```python
from build123d import *

# Parameters (mm, degrees)
SKETCH1_R           = 1
BOSS_EXTRUDE1_DEPTH = 2


with BuildPart() as part:
    # Sketch1 → Boss-Extrude1 (new body)
    with BuildSketch(Plane.XY):
        with BuildLine():
            Line((5.111751732, -19.659180157), (6, -22.203603311))
            ThreePointArc((6, -22.203603311), (0, 23), (-6, -22.203603311))
            Line((-6, -22.203603311), (-5.111751732, -19.659180157))
            ThreePointArc((-5.111751732, -19.659180157), (-5.690422868, -17.488375796), (-7.921535407, -17.224958453))
            ThreePointArc((-7.921535407, -17.224958453), (-10.119267773, -17.659121233), (-12.205757776, -16.843594198))
            ThreePointArc((-12.205757776, -16.843594198), (0, 19), (12.205757776, -16.843594198))
            ThreePointArc((12.205757776, -16.843594198), (10.119267773, -17.659121233), (7.921535407, -17.224958453))
            ThreePointArc((7.921535407, -17.224958453), (5.690422868, -17.488375796), (5.111751732, -19.659180157))
        make_face()
        with Locations((-7, -19)):
            Circle(SKETCH1_R, mode=Mode.SUBTRACT)
        with Locations((7, -19)):
            Circle(SKETCH1_R, mode=Mode.SUBTRACT)
    extrude(amount=BOSS_EXTRUDE1_DEPTH)


solid = part.part
```
Source: CAD feature listing. Evaluate the final solid. Frame: model axes, mm. A direction names the side the tool comes from. Give positions to 0.01 mm unless a question says otherwise; leave off trailing zeros. Loops run counter-clockwise (first coordinate to the right, second up) from the corner with the lowest first, then second, coordinate; pieces in that order, holes last. Notation, with made-up numbers: M -38,55 L -32,55 A13 ccw -32,61 Z; hole C -11,89 d3. An arc over 180 degrees is marked long. Put each result on its own line as item: value.
Q1. Section A-A (y = -6). Return the cut outline in (x, z).
Response values:
outline: M -22.2,0 L -19.36,0 L -19.36,2 L -22.2,2 Z; M 19.36,0 L 22.2,0 L 22.2,2 L 19.36,2 Z
Q2. Mould query, pull axis Y, two halves, no side actions, for faces 4 (the cylindrical face through (-0.696, 18.988, 0.986)), 5 (the flat face through (-5.562, -20.949, 0.986)), 6 (the cylindrical face through (10.151, -17.656, 0.986)), 7 (the flat face through (3, 19, 0)). Classes: released by +Y, released by -Y, zero draft, split by the parting line, or undercut.
Response values:
face 4: undercut
face 5: released by -Y
face 6: undercut
face 7: zero draft
Q3. Section D-D (z = 0.35). Return the cut outline in (x, y), and give its area (3 significant figures).
Response values:
outline: M -12.21,-16.84 A20 cw long 12.21,-16.84 A4 cw 7.92,-17.22 A2 ccw 5.11,-19.66 L 6,-22.2 A23 ccw long -6,-22.2 L -5.11,-19.66 A2 ccw -7.92,-17.22 A4 cw Z; hole C -7,-19 d2; hole C 7,-19 d2
area: 397 mm²
Q4. Line query: probe 1 along Y at (x, z) = (-7, 0.7) (3 decimals); probe 2 along X at (y, z) = (-13.5, 1.35); probe 3 along X at (y, z) = (5, 0.1). Output: solid intervals per line, ascending. Write a range as [from, to].
Response values:
probe 1: y = [-21.909, -20], [-18, -17], [17.735, 21.909]
probe 2: x = [-18.62, -15.61], [15.61, 18.62]
probe 3: x = [-22.45, -19.08], [19.08, 22.45]
Q5. Section B-B (x = -14). Return the cut outline in (y, z), and give its area (3 significant figures).
Response values:
outline: M -18.25,0 L -15.28,0 L -15.28,2 L -18.25,2 Z; M 13.28,0 L 18.25,0 L 18.25,2 L 13.28,2 Z
area: 15.9 mm²
Q6. Pin query (flat end, axial travel): P1, Ø2, axis at x = -1.5, y = 18.5, coming from the +Z side. Return the tip coordinate at first contact, or that it passes through.
Response values:
P1: stops at z = 2
Q7. Reachability of faces 1 (the flat face through (5.55, -20.91, 0.99)), 2 (the flat face through (3, 19, 2)), 3 (the cylindrical face through (-10.09, -17.66, 0.99)) from +Z, -Z, +X, -X, +Y, -Y: full face, straight path, thin tool, end or side. Return the list, or none.
Response values:
face 1: +Z, -Z, -Y
face 2: +Z, +X, -X, +Y, -Y
face 3: +Z, -Z
Q8. Section C-C (x = 7). Return the cut outline in (y, z) (3 decimals).
Response values:
outline: M -21.909,0 L -20,0 L -20,2 L -21.909,2 Z; M -18,0 L -17,0 L -17,2 L -18,2 Z; M 17.735,0 L 21.909,0 L 21.909,2 L 17.735,2 Z
